Work out the finished part from the listing and answer in its coordinate system (mm). A direction names the side the tool comes from. Give positions to 0.01 mm unless a question says otherwise; leave off trailing zeros. Write each loop counter-clockwise with the first axis right and the second up, starting at its lowest first coordinate (ties: lowest second). Pieces come first, ordered by that corner, then holes.
1) Find section D-D (x = -3). Determine the outline of the cut face in (y, z).
2) Straight lines are drawn through the part: probe 1 along Z at (x, y) = (8.5, 17); probe 2 along X at (y, z) = (5.5, -39); probe 3 along Y at (x, z) = (1.5, -41). For each, find the intervals that lie inside material, in ascending order.
3) Find section C-C (x = -31.5). Determine the outline of the cut face in (y, z).
4) Determine the mould class of faces 6 (the face through (-1, 0, 2)), 7 (the face through (-44, 15, 1)) for opening direction X: pulls with the +X half, pulls with the -X half, needs draft (parallel to the pull), parting line crosses it, or undercut.
5) Given pin 1 Ø13 at (y, z) = (-2, -38) entering from -X; pin 2 Ø2 at (x, y) = (-80, -19) entering from -Z; pin 3 Ø10 at (y, z) = (-8, -26) entering from +X, each flat-ended and moving along its own axis, determine where each tip first touches the part or whether it passes through.
6) Find section A-A (x = 83). Determine the outline of the cut face in (y, z).
7) A tool of negligible diameter and unlimited length cuts with its end or side. For faces 1 (the face through (41.5, -5.93, -49.01)), 2 (the face through (-63.57, 2.45, 0.99)), 3 (the face through (48.8, -8.9, 1)), 4 (the face through (73, -1, -24)), 5 (the face through (-81, -20, -20)), from which of +Z, -Z, +X, -X, +Y, -Y can it reach the whole face along a straight path? Write none if from no direction.
8) Find section B-B (z = -18). Determine the outline of the cut face in (x, y).
```python
from build123d import *

# Parameters (mm, degrees)
SKETCH1_W           = 150
SKETCH1_H           = 40
SKETCH1_R           = 9.5
SKETCH1_R_2         = 1.5
BOSS_EXTRUDE1_DEPTH = 2
SKETCH2_W           = 150
SKETCH2_H           = 40
SKETCH2_W_2         = 146
SKETCH2_H_2         = 36
BOSS_EXTRUDE3_DEPTH = 50
CUT_EXTRUDE1_REACH  = 152
SKETCH4_R           = 5
SKETCH8_W           = 146
SKETCH8_H           = 2
CUT_EXTRUDE4_DEPTH  = 48
SKETCH9_W           = 150
SKETCH9_H           = 2
BOSS_EXTRUDE4_DEPTH = 40
SKETCH10_W          = 14
SKETCH10_H          = 2
BOSS_EXTRUDE5_DEPTH = 10
SKETCH11_R          = 2.5
CUT_EXTRUDE5_DEPTH  = 41
SKETCH12_R          = 1.5
SKETCH12_R_2        = 4
CUT_EXTRUDE6_DEPTH  = 2
CUT_EXTRUDE7_DEPTH  = 60
FILLET1_R           = 1


with BuildPart() as part:
    # Sketch1 → Boss-Extrude1 (new body)
    with BuildSketch(Plane.XY):
        Rectangle(SKETCH1_W, SKETCH1_H)
        with Locations((-50, 2)):
            Circle(SKETCH1_R, mode=Mode.SUBTRACT)
        with Locations((-65, 2)):
            Circle(SKETCH1_R_2, mode=Mode.SUBTRACT)
        with Locations((-57.5, 14.990381057)):
            Circle(SKETCH1_R_2, mode=Mode.SUBTRACT)
        with Locations((-42.5, 14.990381057)):
            Circle(SKETCH1_R_2, mode=Mode.SUBTRACT)
        with Locations((-35, 2)):
            Circle(SKETCH1_R_2, mode=Mode.SUBTRACT)
        with Locations((50, -8)):
            Circle(SKETCH1_R_2, mode=Mode.SUBTRACT)
    extrude(amount=BOSS_EXTRUDE1_DEPTH)

    # Sketch2 → Boss-Extrude3 (add)
    with BuildSketch(Plane.XY.offset(2)):
        Rectangle(SKETCH2_W, SKETCH2_H)
        Rectangle(SKETCH2_W_2, SKETCH2_H_2, mode=Mode.SUBTRACT)
    extrude(amount=-BOSS_EXTRUDE3_DEPTH)

    # Sketch4 → Cut-Extrude1 (cut, up to next)
    with BuildSketch(Plane.ZY.offset(75), mode=Mode.PRIVATE) as cut_extrude1_sk1:
        with Locations((-38, -2)):
            Circle(SKETCH4_R)
    cut_extrude1_tool1 = extrude(cut_extrude1_sk1.sketch, amount=-CUT_EXTRUDE1_REACH, mode=Mode.PRIVATE) & part.part
    add(cut_extrude1_tool1.solids().sort_by_distance((-75, -2, -38))[0], mode=Mode.SUBTRACT)

    # Sketch8 → Cut-Extrude4 (cut)
    with BuildSketch(Plane(origin=(0, 0, -48), x_dir=(-1, 0, 0), z_dir=(0, 0, -1))):
        with Locations((0, -19)):
            Rectangle(SKETCH8_W, SKETCH8_H)
    extrude(amount=-CUT_EXTRUDE4_DEPTH, mode=Mode.SUBTRACT)

    # Sketch9 → Boss-Extrude4 (add)
    with BuildSketch(Plane(origin=(0, 20, 0), x_dir=(1, 0, 0), z_dir=(0, 1, 0))):
        with Locations((0, 49)):
            Rectangle(SKETCH9_W, SKETCH9_H)
    extrude(amount=-BOSS_EXTRUDE4_DEPTH)

    # Sketch10 → Boss-Extrude5 (add, symmetric)
    with BuildSketch(Plane.XY.offset(-18)):
        with Locations((-82, -19)):
            Rectangle(SKETCH10_W, SKETCH10_H)
        with Locations((82, -19)):
            Rectangle(SKETCH10_W, SKETCH10_H)
    extrude(amount=BOSS_EXTRUDE5_DEPTH, both=True)

    # Sketch11 → Cut-Extrude5 (cut, through all)
    with BuildSketch(Plane(origin=(0, 20, 0), x_dir=(1, 0, 0), z_dir=(0, 1, 0))):
        with Locations((-83, 18)):
            Circle(SKETCH11_R)
        with Locations((83, 18)):
            Circle(SKETCH11_R)
    extrude(amount=-CUT_EXTRUDE5_DEPTH, mode=Mode.SUBTRACT)

    # Sketch12 → Cut-Extrude6 (cut)
    with BuildSketch(Plane(origin=(0, 0, -50), x_dir=(-1, 0, 0), z_dir=(0, 0, -1))):
        with Locations((-65.004612411, -6)):
            Circle(SKETCH12_R)
        with Locations((-40, -6)):
            Circle(SKETCH12_R)
        with Locations((-5, -6)):
            Circle(SKETCH12_R)
        with Locations((-30.004612411, -6)):
            Circle(SKETCH12_R)
        with Locations((5, -6)):
            Circle(SKETCH12_R_2)
        with BuildLine():
            Line((-59.85474671, -0.512445776), (-45.1498657, -0.512445776))
            ThreePointArc((-45.1498657, -0.512445776), (-43.670729064, -1.166282781), (-43.158706695, -2.700290966))
            Line((-43.158706695, -2.700290966), (-43.781293305, -9.299709034))
            ThreePointArc((-43.781293305, -9.299709034), (-44.426289315, -10.591000482), (-45.772452311, -11.111863845))
            Line((-45.772452311, -11.111863845), (-59.2321601, -11.111863845))
            ThreePointArc((-59.2321601, -11.111863845), (-60.578323096, -10.591000482), (-61.223319106, -9.299709034))
            Line((-61.223319106, -9.299709034), (-61.845905716, -2.700290966))
            ThreePointArc((-61.845905716, -2.700290966), (-61.333883347, -1.166282781), (-59.85474671, -0.512445776))
        make_face()
        with BuildLine():
            Line((-26.845905716, -2.700290966), (-26.223319106, -9.299709034))
            ThreePointArc((-26.223319106, -9.299709034), (-25.578323096, -10.591000482), (-24.2321601, -11.111863845))
            Line((-24.2321601, -11.111863845), (-10.772452311, -11.111863845))
            ThreePointArc((-10.772452311, -11.111863845), (-9.426289315, -10.591000482), (-8.781293305, -9.299709034))
            Line((-8.781293305, -9.299709034), (-8.158706695, -2.700290966))
            ThreePointArc((-8.158706695, -2.700290966), (-8.670729064, -1.166282781), (-10.1498657, -0.512445776))
            Line((-10.1498657, -0.512445776), (-24.85474671, -0.512445776))
            ThreePointArc((-24.85474671, -0.512445776), (-26.333883347, -1.166282781), (-26.845905716, -2.700290966))
        make_face()
    extrude(amount=-CUT_EXTRUDE6_DEPTH, mode=Mode.SUBTRACT)

    # Sketch14 → Cut-Extrude7 (cut)
    with BuildSketch(Plane(origin=(0, 0, -50), x_dir=(-1, 0, 0), z_dir=(0, 0, -1))):
        with BuildLine():
            Line((-75, -20), (75, -20))
            ThreePointArc((75, -20), (0, -16.24057783), (-75, -20))
        make_face()
    extrude(amount=-CUT_EXTRUDE7_DEPTH, mode=Mode.SUBTRACT)

    # Fillet1
    fillet1_edges = [part.edges().sort_by_distance(p)[0] for p in [
        (-75, 0, -50),
        (75, 0, -50),
        (0, 20, -50),
        (-75, 0, 2),
        (75, 0, 2),
        (-75, 20, -24),
        (75, 20, -24),
        (0, 20, 2),
    ]]
    fillet(fillet1_edges, radius=FILLET1_R)


solid = part.part
```
Results:
1. outline: (-16.25, -50) - (-9.46, -50) - (-9.46, -48) - (-16.25, -48) - close; (-16.25, 0) - (18, 0) - (18, -48) - (-2.54, -48) - (-2.54, -50) - (19, -50) arc R1 ccw to (20, -49) - (20, 1) arc R1 ccw to (19, 2) - (-16.25, 2) - close
2. probe 1: z = -50 to -48, 0 to 2
2. probe 2: x = -75 to -73, 73 to 75
2. probe 3: y = 18 to 20
3. outline: (-16.9, -50) - (19, -50) arc R1 ccw to (20, -49) - (20, 1) arc R1 ccw to (19, 2) - (-16.9, 2) - (-16.9, 0) - (18, 0) - (18, -48) - (-16.9, -48) - close
4. face 6: needs draft
4. face 7: undercut
5. pin 1: stops at x = -75
5. pin 2: stops at z = -28
5. pin 3: stops at x = 75
6. outline: (-20, -28) - (-18, -28) - (-18, -20.5) - (-20, -20.5) - close; (-20, -15.5) - (-18, -15.5) - (-18, -8) - (-20, -8) - close
7. face 1: -Z
7. face 2: +Z
7. face 3: +Z, -Z
7. face 4: -Y
7. face 5: +Z, -Z, +X, -X, -Y
8. outline: (-89, -20) - (-85.5, -20) - (-85.5, -18) - (-89, -18) - close; (-80.5, -20) - (-75, -20) arc R750 cw to (-73, -19.8) - (-73, 18) - (73, 18) - (73, -19.8) arc R750 cw to (75, -20) - (80.5, -20) - (80.5, -18) - (75, -18) - (75, 19) arc R1 ccw to (74, 20) - (-74, 20) arc R1 ccw to (-75, 19) - (-75, -18) - (-80.5, -18) - close; (85.5, -20) - (89, -20) - (89, -18) - (85.5, -18) - close
